Here's how the part is built. I have some questions about the finished solid (model axes, mm). Face numbers are marked on the shaded views. Give positions to 0.01 mm unless a question says otherwise; leave off trailing zeros. Order: outer loops, then holes, each group sorted by start corner. A loop starts at its lowest first (then second) coordinate and runs counter-clockwise, first axis right, second up.
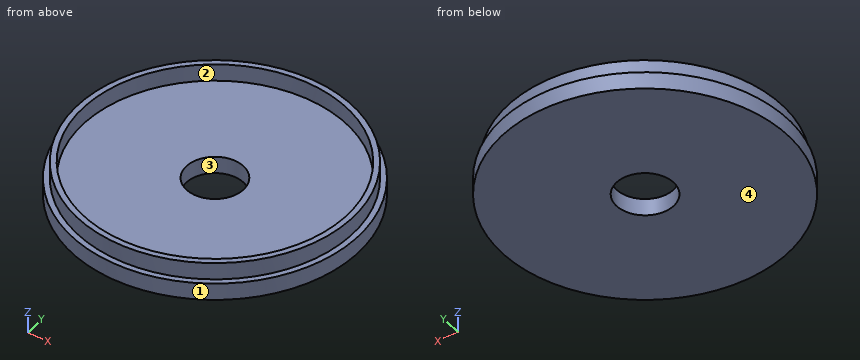
from build123d import *

# Parameters (mm, degrees)
F0_R     = 25
F1_DEPTH = 3
F2_R     = 24
F2_R_2   = 23
F3_DEPTH = 3
F4_D     = 10


with BuildPart() as f1:
    # F0 (on Top) → F1 (new body)
    with BuildSketch(Plane.XY):
        Circle(F0_R)
    extrude(amount=F1_DEPTH)

    # F2 (on face) → F3 (join)
    with BuildSketch(Plane.XY.offset(3)):
        Circle(F2_R)
        Circle(F2_R_2, mode=Mode.SUBTRACT)
    extrude(amount=F3_DEPTH)

    # F4 (through all)
    with Locations(Plane(origin=(0, 0, 0), x_dir=(1, 0, 0), z_dir=(0, 0, -1))):
        with Locations((0, 0)):
            Hole(F4_D / 2)


solid = f1.part
Q1. Thinking about a two-plate mould opening in Y: for the marked faces 1, 2, 3 and 4, which applies, released by +Y, released by -Y, zero draft, split by the parting line, or undercut?
Filled sheet:
face 1: split by the parting line
face 2: undercut
face 3: undercut
face 4: zero draft
Q2. If we section it at A-A on x = 0: List the corners of the cut face in (y, z) for me, plus the area to 3 significant figures.
Filled sheet:
outline: (-25, 0) - (-5, 0) - (-5, 3) - (-23, 3) - (-23, 6) - (-24, 6) - (-24, 3) - (-25, 3) - close; (5, 0) - (25, 0) - (25, 3) - (24, 3) - (24, 6) - (23, 6) - (23, 3) - (5, 3) - close
area: 126 mm2
Q3. I'm going to push flat-ended pins straight in: P1, Ø1, axis at y = 4.5, z = 5, coming from the -X side; P2, Ø1.5, axis at y = -3, z = 1, coming from the -X side; P3, Ø10, axis at x = -1.5, y = -7.5, coming from the +Z side; P4, Ø8, axis at x = 0, y = 0, coming from the -Z side. Where does each tip first touch, or does it pass through?
Filled sheet:
P1: stops at x = -23.66
P2: stops at x = -24.9
P3: stops at z = 3
P4: passes through
Q4. I need wall thicknesses on L1, parallel to Y at x = 0, z = 2.3; L2, parallel to Y at x = 0, z = 3.95; L3, parallel to Z at x = -14, y = 11.5. Which ranges of each line are inside material? Lowest first, please.
Filled sheet:
L1: y = -25 to -5, 5 to 25
L2: y = -24 to -23, 23 to 24
L3: z = 0 to 3
Q5. If we section it at C-C on z = 3.75: List the corners of the cut face in (x, y) for me, plus the area to 3 significant figures.
Filled sheet:
outline: circle Ø48 at (0, 0); hole circle Ø46 at (0, 0)
area: 148 mm2
Q6. If we section it at D-D on x = 17.5: List the corners of the cut face in (y, z) for me.
Filled sheet:
outline: (-17.85, 0) - (17.85, 0) - (17.85, 3) - (16.42, 3) - (16.42, 6) - (14.92, 6) - (14.92, 3) - (-14.92, 3) - (-14.92, 6) - (-16.42, 6) - (-16.42, 3) - (-17.85, 3) - close
